from build123d import *

# Parameters (mm, degrees)
SKETCH1_W               = 19.05
SKETCH1_H               = 19.05
SKETCH1_W_2             = 15.875
SKETCH1_H_2             = 15.875
BOSS_EXTRUDE1_DEPTH     = 406.4
CUT_EXTRUDE1_DEPTH      = 407.623180906
CUT_EXTRUDE1_DEPTH_BACK = 407.623180906
SKETCH2_R               = 2.38125


with BuildPart() as part:
    # Sketch1 → Boss-Extrude1 (new body)
    with BuildSketch(Plane.XY):
        Rectangle(SKETCH1_W, SKETCH1_H)
        Rectangle(SKETCH1_W_2, SKETCH1_H_2, mode=Mode.SUBTRACT)
    extrude(amount=BOSS_EXTRUDE1_DEPTH)

    # Sketch2 → Cut-Extrude1 (cut, two sides: drawn at the far end of the back side and taken through both)
    with BuildSketch(Plane(origin=(0, 0, 0), x_dir=(1, 0, 0), z_dir=(0, 1, 0)).offset(-CUT_EXTRUDE1_DEPTH_BACK)):
        with Locations(Location((0, -12.7, 0), (0, 0, 270))):
            Circle(SKETCH2_R)
        with Locations(Location((0, -63.5, 0), (0, 0, 270))):
            Circle(SKETCH2_R)
    extrude(amount=CUT_EXTRUDE1_DEPTH + CUT_EXTRUDE1_DEPTH_BACK, mode=Mode.SUBTRACT)


solid = part.part
The listing builds one solid part. Answer for the finished solid, in the listing's coordinates (mm). A direction names the side the tool comes from. Coordinates: 2 decimals unless noted, no trailing zeros. Order: outer loops, then holes, each group sorted by start corner. A loop starts at its lowest first (then second) coordinate and runs counter-clockwise, first axis right, second up. Notation, with made-up numbers: (-8, 13) -> (2, 13) arc R14 cw to (2, 25) -> close; hole circle Ø7 at (-6.75, 76.5). An arc over 180 degrees is marked (long way). Answer in a Markdown table with one row per item. Add a question column.
Item 1: Find section A-A (y = -0.75). Write down the section's boundary in (x, z) (1 decimal).
Item 2: Find the intervals of material crossed by L1, parallel to Z at x = 0, y = -9; L2, parallel to Y at x = -2.5, z = 143 (1 decimal), in increasing order. Write a range as from..to.
Item 3: Determine the mould class of faces 1 (the face through (0, -9.525, 200)), 2 (the face through (-9.525, 0, 200)), 3 (the face through (-7.938, 0, 200)) for opening direction X: +X half, -X half, draft (parallel to the pull), parting line (faces both ways), or undercut.
Item 4: Which of the six approach directions +Z, -Z, +X, -X, +Y, -Y give full straight-line access (tool end or side, diameter ignored) to faces 4 (the face through (0, 9.525, 200)), 5 (the face through (7.938, 0, 200))?
Item 5: Find section B-B (z = 341.5). Write down the section's boundary in (x, y) (1 decimal).
Result set:
| question | item | result |
|---|---|---|
| 1 | outline | (-9.5, 0) -> (-7.9, 0) -> (-7.9, 406.4) -> (-9.5, 406.4) -> close; (7.9, 0) -> (9.5, 0) -> (9.5, 406.4) -> (7.9, 406.4) -> close |
| 2 | L1 | z = 0..10.32, 15.08..61.12, 65.88..406.4 |
| 2 | L2 | y = -9.5..-7.9, 7.9..9.5 |
| 3 | face 1 | draft |
| 3 | face 2 | -X half |
| 3 | face 3 | undercut |
| 4 | face 4 | +Z, -Z, +X, -X, +Y |
| 4 | face 5 | +Z, -Z |
| 5 | outline | (-9.5, -9.5) -> (9.5, -9.5) -> (9.5, 9.5) -> (-9.5, 9.5) -> close; hole (-7.9, -7.9) -> (7.9, -7.9) -> (7.9, 7.9) -> (-7.9, 7.9) -> close |
